```python
from build123d import *

# Parameters (mm, degrees)
F1_DEPTH = 63.5
F2_DEPTH = 21.082
F3_DEPTH = 48.006


# Not quite as in the source:
# - a feature of the source that left no trace in its solid (it failed there, or was rolled back) is left out


with BuildPart() as f1:
    # F0 (on Front) → F1 (new body, symmetric)
    with BuildSketch(Plane.XZ):
        Polygon((0, -27.6409685612), (0, 0), (-8.890000172, 0), (-49.0482896566, 0), (-49.0482896566, -27.6409685612), align=None)
    extrude(amount=F1_DEPTH, both=True)

    # F0 (on Front) → F2 (join, symmetric)
    with BuildSketch(Plane.XZ):
        with BuildLine():
            Line((-8.890000172, 0), (0, 0))
            Line((0, 0), (0, 28.5326149315))
            ThreePointArc((0, 28.5326149315), (-10.4057051367, 39.6136101279), (2.7482079064, 47.2321221605))
            Line((2.7482079064, 47.2321221605), (32.5638093054, 47.2321221605))
            Line((32.5638093054, 47.2321221605), (32.5638093054, 56.1221223325))
            Line((32.5638093054, 56.1221223325), (4.1557957579, 56.1221223325))
            ThreePointArc((4.1557957579, 56.1221223325), (-18.2071887125, 44.7519974591), (-8.890000172, 21.4588050682))
            Line((-8.890000172, 21.4588050682), (-8.890000172, 0))
        make_face()
    extrude(amount=F2_DEPTH, both=True)

    # F0 (on Front) → F3 (join, symmetric)
    with BuildSketch(Plane.XZ):
        Polygon((32.5638093054, 56.1221223325), (32.5638093054, 47.2321221605), (32.5638093054, 34.5321221605), (59.3218803406, 34.5321221605), (59.3218803406, 59.9321221605), (32.5638093054, 59.9321221605), align=None)
    extrude(amount=F3_DEPTH, both=True)


solid = f1.part
```
Can you work these out from the model? Positions are in its coordinate system, mm. A direction names the side the tool comes from. Give positions to 0.01 mm unless a question says otherwise; leave off trailing zeros. Loops run counter-clockwise (first coordinate to the right, second up) from the corner with the lowest first, then second, coordinate; pieces in that order, holes last. Notation, with made-up numbers: M -7,40.5 L 49,40.5 A5 cw 49,49.5 Z; hole C 37.25,58 d4. An arc over 180 degrees is marked long. Answer in a Markdown table with one row per item.
1. Which directions (+Z, -Z, +X, -X, +Y, -Y) give clear straight access to the entire face, cutting with the end or side of a thin tool? Please do faces 4 (the flat face through (-8.89, 0, 11)), 5 (the flat face through (2.6, 21.082, 47.5)), 6 (the flat face through (2.6, -21.082, 47.5)).
Taken from the geometry:
| item | result |
|---|---|
| face 4 | -X, +Y, -Y |
| face 5 | +Z, -X, +Y |
| face 6 | +Z, -X, -Y |
2. Suppose I cut it at A-A on y = -30.5. Write out the boundary of the cut face in (x, z).
Taken from the geometry:
| item | result |
|---|---|
| outline | M -49.05,-27.64 L 0,-27.64 L 0,0 L -49.05,0 Z; M 32.56,34.53 L 59.32,34.53 L 59.32,59.93 L 32.56,59.93 Z |
3. Suppose I cut it at B-B on x = 50. Write out the boundary of the cut face in (y, z).
Taken from the geometry:
| item | result |
|---|---|
| outline | M -48.01,34.53 L 48.01,34.53 L 48.01,59.93 L -48.01,59.93 Z |
4. Suppose I cut it at C-C on z = -19. Write out the boundary of the cut face in (x, y), plus the area to 3 significant figures.
Taken from the geometry:
| item | result |
|---|---|
| outline | M -49.05,-63.5 L 0,-63.5 L 0,63.5 L -49.05,63.5 Z |
| area | 6,230 mm² |
5. For pin 1 Ø8 at (y, z) = (-1, 10.5) entering from -X; pin 2 Ø21.5 at (x, y) = (44, -17) entering from -Z; pin 3 Ø12.5 at (x, z) = (48.5, 42.5) entering from +Y; pin 4 Ø11.5 at (x, z) = (-0.81, 38.2) entering from -Y, each with a flat end and sliding along its axis, tell me the tip position at first contact or that it passes through.
Taken from the geometry:
| item | result |
|---|---|
| pin 1 | stops at x = -8.89 |
| pin 2 | stops at z = 34.53 |
| pin 3 | stops at y = 48.01 |
| pin 4 | passes through |
6. If I drill on line 1 along X through (y, z) = (26.5, 45); line 2 along X through (y, z) = (25, -1.5); line 3 along Z through (x, y) = (-33, -17.5), over which ranges is the centre line in solid material (lowest first)?
Taken from the geometry:
| item | result |
|---|---|
| line 1 | x = 32.56 to 59.32 |
| line 2 | x = -49.05 to 0 |
| line 3 | z = -27.64 to 0 |
7. Thinking about a two-plate mould opening in X: for faces 1 (the flat face through (0, -1, -6)), 2 (the flat face through (-25, -1, -27.641)), 3 (the cylindrical face through (-10.44, -0.3, 39.37)), which applies, released by +X, released by -X, zero draft, split by the parting line, or undercut?
Taken from the geometry:
| item | result |
|---|---|
| face 1 | released by +X |
| face 2 | zero draft |
| face 3 | undercut |
